Geometry check sheet. Reference: the model listing, model coordinates, mm. A direction names the side the tool comes from. Coordinates: 2 decimals unless noted, no trailing zeros. Put each result on its own line as item: value. Start each with the question number.
1) Mould release check, pull along X, two halves, no side actions. Record for faces 4 (the flat face through (32.14, -122.58, 5.45)), 5 (the cylindrical face through (14.58, -1.93, 8.54)), 6 (the flat face through (-20, -70, 11)), 7 (the cylindrical face through (0, -255, 5)): released by +X, released by -X, zero draft, split by the parting line, or undercut.
2) Gauge pin test, flat ends, axial feed: pin 1 (5 mm diameter, centred on x = -16.79, y = 3.96, fed in from +Z); pin 2 (6 mm diameter, centred on y = -95, z = 8, fed in from +X); pin 3 (3 mm diameter, centred on y = -67.5, z = 6.5, fed in from -X). Record the tip position at first contact, or that the pin passes through.
3) Set-up check for faces 1 (the cylindrical face through (31.92, -119.27, 10.4)), 2 (the flat face through (-12.56, -130.66, 5.42)), 3 (the flat face through (19, -5, 6)): record each of +Z, -Z, +X, -X, +Y, -Y from which the full face is reachable in a straight line by a thin tool's end or side.
4) Scan lines: line 1 along X through (y, z) = (-74, 5.75); line 2 along X through (y, z) = (-127.5, 1.5); line 3 along X through (y, z) = (-224, 5.5). Record each from-to range of solid material in increasing order.
from build123d import *

# Parameters (mm, degrees)
EXTRUDE_1_DEPTH     = 11
SKETCH_2_R          = 10
CUT_EXTRUDE_1_DEPTH = 11
FILLET_1_R          = 2
CUT_EXTRUDE_2_DEPTH = 20
SKETCH_6_R          = 2
CUT_EXTRUDE_4_DEPTH = 33
SKETCH_7_R          = 3
CUT_EXTRUDE_5_DEPTH = 5


with BuildPart() as part:
    # 草图1 → 凸台-拉伸1 (new body)
    with BuildSketch(Plane.XY):
        with BuildLine():
            Line((-44.744635323, -4.787234043), (-19.886504588, -237.127659574))
            ThreePointArc((-19.886504588, -237.127659574), (0, -255), (19.886504588, -237.127659574))
            Line((19.886504588, -237.127659574), (44.744635323, -4.787234043))
            ThreePointArc((44.744635323, -4.787234043), (0, 45), (-44.744635323, -4.787234043))
        make_face()
    extrude(amount=EXTRUDE_1_DEPTH)

    # 草图2 → 切除-拉伸1 (cut)
    with BuildSketch(Plane(origin=(0, 0, 0), x_dir=(-1, 0, 0), z_dir=(0, 0, -1))):
        with Locations((0, -235.836034695)):
            Circle(SKETCH_2_R)
    extrude(amount=-CUT_EXTRUDE_1_DEPTH, mode=Mode.SUBTRACT)

    # 圆角1
    fillet_1_edges = [part.edges().sort_by_distance(p)[0] for p in [
        (0, -255, 11),
        (32.315569956, -120.957446809, 11),
        (0, 45, 11),
        (32.315569956, -120.957446809, 0),
        (0, -255, 0),
        (-32.315569956, -120.957446809, 0),
        (0, 45, 0),
        (-32.315569956, -120.957446809, 11),
    ]]
    fillet(fillet_1_edges, radius=FILLET_1_R)

    # 草图4 → 切除-拉伸2 (cut)
    with BuildSketch(Plane(origin=(0, 0, 0), x_dir=(-1, 0, 0), z_dir=(0, 0, -1))):
        with BuildLine():
            Line((-21.759824224, -44.682312886), (-3.625991278, -214.173032358))
            ThreePointArc((-3.625991278, -214.173032358), (0.015295132, -212.723088949), (3.615338262, -214.272602446))
            Line((3.615338262, -214.272602446), (21.759824224, -44.682312886))
            ThreePointArc((21.759824224, -44.682312886), (0, -50.060383894), (-21.759824224, -44.682312886))
        make_face()
    extrude(amount=-CUT_EXTRUDE_2_DEPTH, mode=Mode.SUBTRACT)

    # 草图6 → 切除-拉伸4 (cut)
    with BuildSketch(Plane.XY.offset(11)):
        with Locations((-16.789244382, 3.960274368)):
            Circle(SKETCH_6_R)
        with Locations((-4.964923982, 16.52004933)):
            Circle(SKETCH_6_R)
        with Locations((11.8243204, 12.559774961)):
            Circle(SKETCH_6_R)
        with Locations((16.789244382, -3.960274368)):
            Circle(SKETCH_6_R)
        with Locations((4.964923982, -16.52004933)):
            Circle(SKETCH_6_R)
        with Locations((-11.8243204, -12.559774961)):
            Circle(SKETCH_6_R)
    extrude(amount=-CUT_EXTRUDE_4_DEPTH, mode=Mode.SUBTRACT)

    # 草图7 → 切除-拉伸5 (cut)
    with BuildSketch(Plane.XY.offset(11)):
        with Locations((-4.964923982, 16.52004933)):
            Circle(SKETCH_7_R)
        with Locations((11.8243204, 12.559774961)):
            Circle(SKETCH_7_R)
        with Locations((16.789244382, -3.960274368)):
            Circle(SKETCH_7_R)
        with Locations((4.964923982, -16.52004933)):
            Circle(SKETCH_7_R)
        with Locations((-11.8243204, -12.559774961)):
            Circle(SKETCH_7_R)
        with Locations((-16.789244382, 3.960274368)):
            Circle(SKETCH_7_R)
    extrude(amount=-CUT_EXTRUDE_5_DEPTH, mode=Mode.SUBTRACT)


solid = part.part
Answer key:
1. face 4: released by +X
1. face 5: undercut
1. face 6: zero draft
1. face 7: split by the parting line
2. pin 1: stops at z = 6
2. pin 2: stops at x = 35.41
2. pin 3: stops at x = -38.2
3. face 1: +Z, +X, -Y
3. face 2: +Z, -Z
3. face 3: +Z
4. line 1: x = -37.34 to -18.62, 18.62 to 37.34
4. line 2: x = -31.55 to -12.9, 12.9 to 31.55
4. line 3: x = -21.29 to 21.29
